Print and shaded views of the part. All mm, measured from the part's lowest x, y and z. A direction names the side the tool comes from. Coordinates: 2 decimals unless noted, no trailing zeros. Loops run counter-clockwise (first coordinate to the right, second up) from the corner with the lowest first, then second, coordinate; pieces in that order, holes last. Notation, with made-up numbers: M -38,14 L -13,14 A21 cw -13,19 Z; hole C -35,-22.5 d8. An arc over 180 degrees is marked long. Use a Markdown table: item, result. Add a question column.
1) Band-saw the part on B-B (x = 2.45). List the corners of the cut face in (y, z).
2) Wall check: probe 1 along X at (y, z) = (1.75, 5); probe 2 along Y at (x, z) = (4.2, 4.25); probe 3 along Z at (x, y) = (5.4, 1.75). Give the ranges that are in metal, low to high. Write a range as from..to.
3) Band-saw the part on D-D (x = 5.5). List the corners of the cut face in (y, z).
4) Pull direction X, two halves, no side cores. Call the marked faces 4, 5 and 6: released by +X, released by -X, zero draft, split by the parting line, or undercut.
5) Pin check, flat tips, straight feed: pin 1 Ø1.9 at (y, z) = (8, 3.5) entering from -X; pin 2 Ø2.5 at (y, z) = (8.5, 2.5) entering from +X; pin 3 Ø1.9 at (x, y) = (3.5, 8.5) entering from -Z. Stop position of each tip, or through.
6) Band-saw the part on A-A (z = 3). List the corners of the cut face in (x, y), plus the area to 3 significant figures.
7) Tool access for the marked faces 1, 2 and 3: list every direction of +Z, -Z, +X, -X, +Y, -Y with a clear straight run to the whole face (end or side of a thin tool).
8) Band-saw the part on C-C (z = 1). List the corners of the cut face in (x, y).
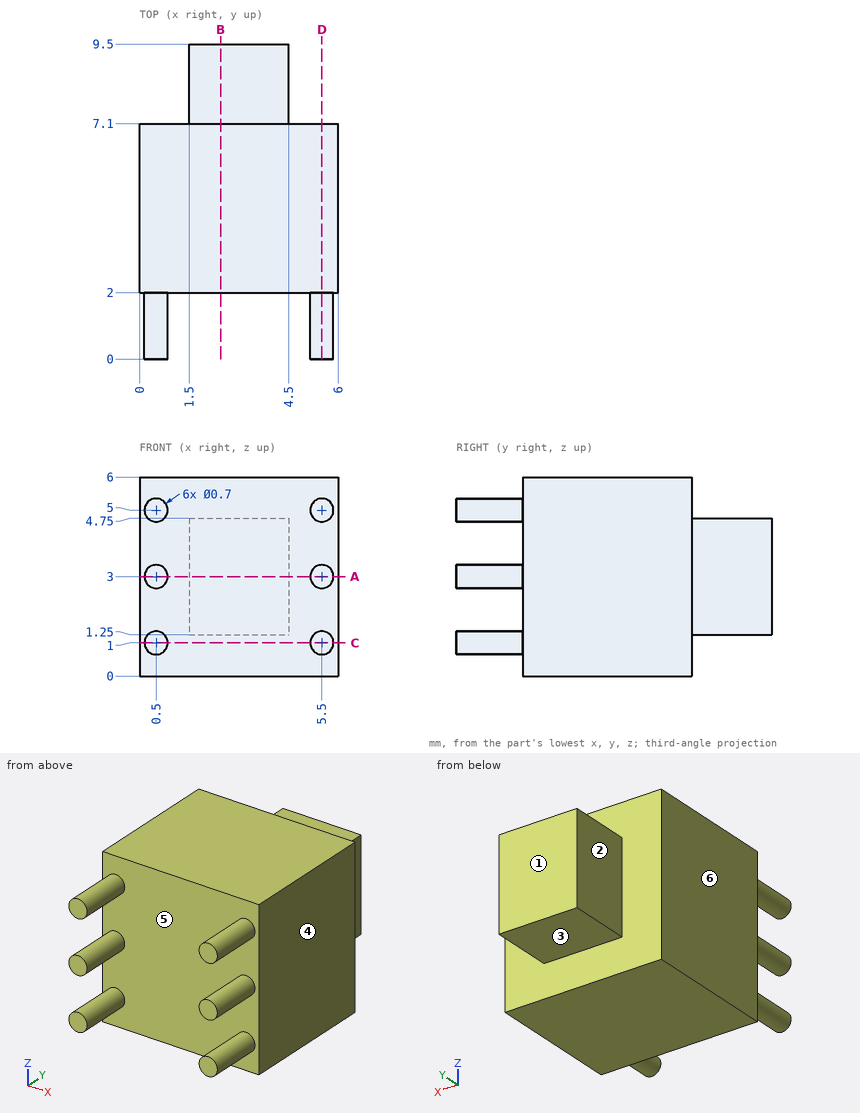
Entries:
| question | item | result |
|---|---|---|
| 1 | outline | M 2,0 L 7.1,0 L 7.1,1.25 L 9.5,1.25 L 9.5,4.75 L 7.1,4.75 L 7.1,6 L 2,6 Z |
| 2 | probe 1 | 0.15..0.85, 5.15..5.85 |
| 2 | probe 2 | 2..9.5 |
| 2 | probe 3 | 0.66..1.34, 2.66..3.34, 4.66..5.34 |
| 3 | outline | M 0,0.65 L 2,0.65 L 2,0 L 7.1,0 L 7.1,6 L 2,6 L 2,5.35 L 0,5.35 L 0,4.65 L 2,4.65 L 2,3.35 L 0,3.35 L 0,2.65 L 2,2.65 L 2,1.35 L 0,1.35 Z |
| 4 | face 4 | released by +X |
| 4 | face 5 | undercut |
| 4 | face 6 | released by -X |
| 5 | pin 1 | x = 0 |
| 5 | pin 2 | x = 4.5 |
| 5 | pin 3 | z = 1.25 |
| 6 | outline | M 0,2 L 0.15,2 L 0.15,0 L 0.85,0 L 0.85,2 L 5.15,2 L 5.15,0 L 5.85,0 L 5.85,2 L 6,2 L 6,7.1 L 4.5,7.1 L 4.5,9.5 L 1.5,9.5 L 1.5,7.1 L 0,7.1 Z |
| 6 | area | 40.6 mm2 |
| 7 | face 1 | +Z, -Z, +X, -X, +Y |
| 7 | face 2 | +Z, -Z, -X, +Y |
| 7 | face 3 | -Z, +X, -X, +Y |
| 8 | outline | M 0,2 L 0.15,2 L 0.15,0 L 0.85,0 L 0.85,2 L 5.15,2 L 5.15,0 L 5.85,0 L 5.85,2 L 6,2 L 6,7.1 L 0,7.1 Z |
